For this review, use the dimensioned drawing (mm, ordinates from the lowest corner) and the shaded views. A direction names the side the tool comes from. Coordinates: 2 decimals unless noted, no trailing zeros. Write each loop counter-clockwise with the first axis right and the second up, starting at its lowest first coordinate (ties: lowest second). Pieces come first, ordered by that corner, then holes.
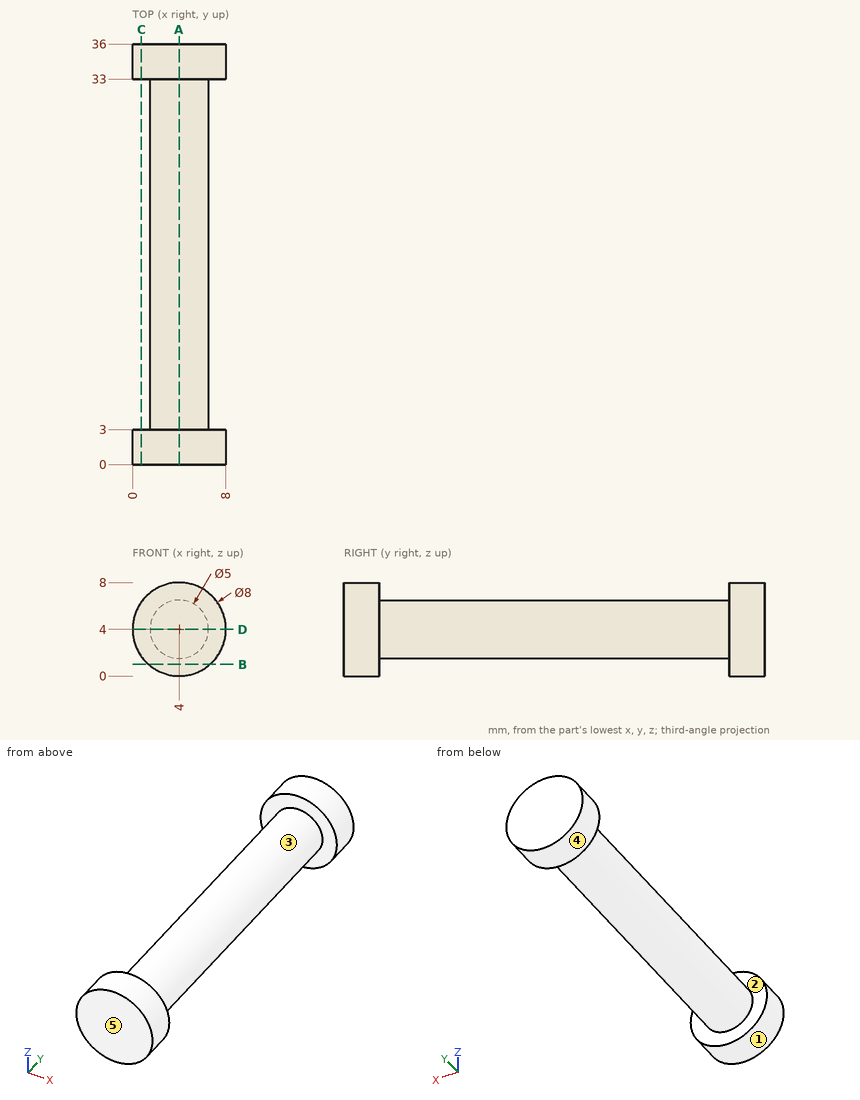
Item 1: To check wall thickness, follow line 1 along Y through (x, z) = (1, 3.75); line 2 along Z through (x, y) = (4, 14.5); line 3 along X through (y, z) = (26, 5). State the ranges of each line that lie inside material, in increasing order.
Solved:
line 1: y = 0 to 3, 33 to 36
line 2: z = 1.5 to 6.5
line 3: x = 1.71 to 6.29
Item 2: Mouldability with a two-part tool opening along Y and no side actions: class the marked faces 3, 4 and 5 as pulls with the +Y half, pulls with the -Y half, needs draft (parallel to the pull), parting line crosses it, or undercut.
Solved:
face 3: undercut
face 4: needs draft
face 5: pulls with the -Y half
Item 3: Take a section at B-B, the plane z = 1. Write out the cut boundary in (x, y), plus the area to 3 significant figures.
Solved:
outline: (1.35, 0) - (6.65, 0) - (6.65, 3) - (1.35, 3) - close; (1.35, 33) - (6.65, 33) - (6.65, 36) - (1.35, 36) - close
area: 31.7 mm2
Item 4: Take a section at C-C, the plane x = 0.75. Write out the cut boundary in (y, z), plus the area to 3 significant figures.
Solved:
outline: (0, 1.67) - (3, 1.67) - (3, 6.33) - (0, 6.33) - close; (33, 1.67) - (36, 1.67) - (36, 6.33) - (33, 6.33) - close
area: 28.0 mm2
Item 5: Take a section at A-A, the plane x = 4. Write out the cut boundary in (y, z).
Solved:
outline: (0, 0) - (3, 0) - (3, 1.5) - (33, 1.5) - (33, 0) - (36, 0) - (36, 8) - (33, 8) - (33, 6.5) - (3, 6.5) - (3, 8) - (0, 8) - close
Item 6: Take a section at D-D, the plane z = 4. Write out the cut boundary in (x, y).
Solved:
outline: (0, 0) - (8, 0) - (8, 3) - (6.5, 3) - (6.5, 33) - (8, 33) - (8, 36) - (0, 36) - (0, 33) - (1.5, 33) - (1.5, 3) - (0, 3) - close
Item 7: For pin 1 (1.5 mm diameter, centred on y = 30.5, z = 6, fed in from -X); pin 2 (3 mm diameter, centred on x = 4.5, y = 13, fed in from +Z); pin 3 (1.5 mm diameter, centred on x = 6.5, y = 15, fed in from +Z), all flat-tipped, find the tip position at first contact; note any pin that passes through.
Solved:
pin 1: stops at x = 1.83
pin 2: stops at z = 6.5
pin 3: stops at z = 5.79
Item 8: Machinability: for the marked faces 1 and 2, which of the approach directions +Z, -Z, +X, -X, +Y, -Y give a long, thin tool a straight path to every point of the face, cutting with its end or side? Answer none if there is none.
Solved:
face 1: +Y, -Y
face 2: none
